from build123d import *

# Parameters (mm, degrees)
F0_R      = 26.924
F1_DEPTH  = 16.764
F0_R_2    = 27.94
F2_DEPTH  = 16.002
F0_R_3    = 22.225
F3_DEPTH  = 5.08
F4_SIZE   = 1.016
F0_W      = 3.175
F0_H      = 1.016
F5_DEPTH  = 23.622
F7_DEPTH  = 1.5875
F8_COUNT  = 3
F9_COUNT  = 2
F9_ANGLE  = 30
F10_COUNT = 3


with BuildPart() as f1:
    # F0 (on Top) → F1 (new body)
    with BuildSketch(Plane.XY):
        Circle(F0_R)
        with BuildLine():
            ThreePointArc((1.5875, 25.3503420835), (18.5132722661, 17.3901912008), (25.4, 0))
            ThreePointArc((25.4, 0), (-17.3901912008, -18.5132722661), (-1.5875, 25.3503420835))
            Line((-1.5875, 25.3503420835), (-1.5875, 25.908))
            Line((-1.5875, 25.908), (1.5875, 25.908))
            Line((1.5875, 25.908), (1.5875, 25.3503420835))
        make_face(mode=Mode.SUBTRACT)
        with BuildLine():
            ThreePointArc((-1.5875, 25.3503420835), (0, 25.4), (1.5875, 25.3503420835))
            Line((1.5875, 25.3503420835), (1.5875, 25.908))
            Line((1.5875, 25.908), (-1.5875, 25.908))
            Line((-1.5875, 25.908), (-1.5875, 25.3503420835))
        make_face()
    extrude(amount=F1_DEPTH)

    # F0 (on Top) → F2 (join)
    with BuildSketch(Plane.XY):
        Circle(F0_R_2)
        Circle(F0_R, mode=Mode.SUBTRACT)
    extrude(amount=F2_DEPTH)

    # F0 (on Top) → F3 (join)
    with BuildSketch(Plane.XY):
        with BuildLine():
            Line((1.5875, 24.892), (1.5875, 25.3503420835))
            ThreePointArc((1.5875, 25.3503420835), (0, 25.4), (-1.5875, 25.3503420835))
            Line((-1.5875, 25.3503420835), (-1.5875, 24.892))
            Line((-1.5875, 24.892), (1.5875, 24.892))
        make_face()
        with BuildLine():
            ThreePointArc((-1.5875, 25.3503420835), (-17.3901912008, -18.5132722661), (25.4, 0))
            ThreePointArc((25.4, 0), (18.5132722661, 17.3901912008), (1.5875, 25.3503420835))
            Line((1.5875, 25.3503420835), (1.5875, 24.892))
            Line((1.5875, 24.892), (1.5875, 23.876))
            Line((1.5875, 23.876), (-1.5875, 23.876))
            Line((-1.5875, 23.876), (-1.5875, 24.892))
            Line((-1.5875, 24.892), (-1.5875, 25.3503420835))
        make_face()
        Circle(F0_R_3, mode=Mode.SUBTRACT)
    extrude(amount=F3_DEPTH)

    # F4
    f4_edges = [f1.edges().sort_by_distance(p)[0] for p in [
        (-27.94, 0, 0),
        (-22.225, 0, 0),
    ]]
    chamfer(f4_edges, length=F4_SIZE)

    # F0 (on Top) → F5 (join)
    with BuildSketch(Plane.XY):
        with BuildLine():
            ThreePointArc((-1.5875, 25.3503420835), (0, 25.4), (1.5875, 25.3503420835))
            Line((1.5875, 25.3503420835), (1.5875, 25.908))
            Line((1.5875, 25.908), (-1.5875, 25.908))
            Line((-1.5875, 25.908), (-1.5875, 25.3503420835))
        make_face()
        with BuildLine():
            Line((1.5875, 24.892), (1.5875, 25.3503420835))
            ThreePointArc((1.5875, 25.3503420835), (0, 25.4), (-1.5875, 25.3503420835))
            Line((-1.5875, 25.3503420835), (-1.5875, 24.892))
            Line((-1.5875, 24.892), (1.5875, 24.892))
        make_face()
        with Locations((0, 24.384)):
            Rectangle(F0_W, F0_H)
    extrude(amount=F5_DEPTH)

    # F6 (on Right) → F7 (join, symmetric)
    with BuildSketch(Plane.YZ):
        Polygon((25.908, 20.8915), (27.94, 20.8915), (25.908, 23.622), align=None)
    extrude(amount=F7_DEPTH, both=True)

    # F8: F1 ×3 about axis
    f8_axis = Axis((0, 0, 10.7297506183), (0, 0, 1))


with BuildPart() as f1_1:
    add(f1.part)
    for i in range(1, F8_COUNT):
        add(f1.part.rotate(f8_axis, i * 360 / F8_COUNT))

    # F9: F1 ×2 about axis
    f9_axis = Axis((0, 0, 10.7297506183), (0, 0, 1))


with BuildPart() as f1_2:
    add(f1_1.part)
    for i in range(1, F9_COUNT):
        add(f1_1.part.rotate(f9_axis, i * F9_ANGLE / (F9_COUNT - 1)))

    # F10: F1 ×3 about axis
    f10_axis = Axis((0, 0, 10.7297506183), (0, 0, 1))


with BuildPart() as f1_3:
    add(f1_2.part)
    for i in range(1, F10_COUNT):
        add(f1_2.part.rotate(f10_axis, i * 360 / F10_COUNT))


solid = f1_3.part
Can you work these out from the model? Positions are in its coordinate system, mm. A direction names the side the tool comes from. Give positions to 0.01 mm unless a question says otherwise; leave off trailing zeros. Order: outer loops, then holes, each group sorted by start corner. A loop starts at its lowest first (then second) coordinate and runs counter-clockwise, first axis right, second up. Notation, with made-up numbers: (50.5, 44.25) - (64.5, 44.25) arc R31 ccw to (64.5, 73.25) - close; hole circle Ø8 at (-30, -28). An arc over 180 degrees is marked (long way). Write each question's results on one line, items separated by ' | '.
1) Please list where these lines run through material, in increasing order: line 1 along Y through (x, z) = (0, 4.35) (3 decimals); line 2 along X through (y, z) = (20, 9.25); line 3 along Z through (x, y) = (21.5, 15). Write a range as [from, to].
Final values:
line 1: y = [-27.94, -22.225], [22.225, 27.94] | line 2: x = [-19.51, -15.66], [-13.38, -13.11], [15.66, 19.51] | line 3: z = [0, 16.76]
2) If we mould it in two halves opening along Y, with no side actions, what happens to faces 1 (the face through (23, -13, 20.892)), 2 (the face through (-22.45, -12.93, 18.8)), 3 (the face through (-0.1, -22.5, 5.08))? For each: pulls with the +Y half, pulls with the -Y half, needs draft (parallel to the pull), parting line crosses it, or undercut.
Final values:
face 1: needs draft | face 2: pulls with the -Y half | face 3: undercut
3) Suppose I cut it at B-B, the plane z = 18.25. Write out the boundary of the cut face in (x, y).
Final values:
outline: (-23.23, -11.58) - (-21.64, -14.33) - (-19.88, -13.31) - (-21.47, -10.56) - close; (-14.33, -21.64) - (-11.58, -23.23) - (-10.56, -21.47) - (-13.31, -19.88) - close; (-14.33, 21.64) - (-13.31, 19.88) - (-10.56, 21.47) - (-11.58, 23.23) - close; (-1.59, 23.88) - (1.59, 23.88) - (1.59, 25.91) - (-1.59, 25.91) - close; (19.88, -13.31) - (21.64, -14.33) - (23.23, -11.58) - (21.47, -10.56) - close; (23.88, -1.59) - (25.91, -1.59) - (25.91, 1.59) - (23.88, 1.59) - close
4) On a 3-axis mill with a long thin cutter (end or side, diameter ignored), from which of +Z, -Z, +X, -X, +Y, -Y can I reach the whole of each face in a straight line? I mean faces 4 (the face through (21.199, 6.676, 3.02)), 5 (the face through (-11.1, 22.4, 16.5)). Say none if no direction works.
Final values:
face 4: +Z, -Z | face 5: +Z
5) Suppose I cut it at D-D, the plane z = 15. Write out the boundary of the cut face in (x, y), then the cut area to 3 significant figures.
Final values:
outline: circle Ø55.88 at (0, 0); hole (-22.75, -11.3) - (-21.47, -10.56) - (-19.88, -13.31) - (-21.16, -14.05) arc R25.4 ccw to (-14.05, -21.16) - (-13.31, -19.88) - (-10.56, -21.47) - (-11.3, -22.75) arc R25.4 ccw to (21.16, -14.05) - (19.88, -13.31) - (21.47, -10.56) - (22.75, -11.3) arc R25.4 ccw to (25.35, -1.59) - (23.88, -1.59) - (23.88, 1.59) - (25.35, 1.59) arc R25.4 ccw to (1.59, 25.35) - (1.59, 23.88) - (-1.59, 23.88) - (-1.59, 25.35) arc R25.4 ccw to (-11.3, 22.75) - (-10.56, 21.47) - (-13.31, 19.88) - (-14.05, 21.16) arc R25.4 ccw to start | area: 454 mm^2
6) Suppose I cut it at A-A, the plane x = 0. Write out the boundary of the cut face in (y, z) (1 decimal).
Final values:
outline: (-27.9, 1) - (-26.9, 0) - (-23.2, 0) - (-22.2, 1) - (-22.2, 5.1) - (-25.4, 5.1) - (-25.4, 16.8) - (-26.9, 16.8) - (-26.9, 16) - (-27.9, 16) - close; (22.2, 1) - (23.2, 0) - (26.9, 0) - (27.9, 1) - (27.9, 16) - (26.9, 16) - (26.9, 16.8) - (25.9, 16.8) - (25.9, 20.9) - (27.9, 20.9) - (25.9, 23.6) - (23.9, 23.6) - (23.9, 5.1) - (22.2, 5.1) - close
7) I'm going to push flat-ended pins straight in: pin 1 Ø8 at (y, z) = (-2, 15) entering from +X; pin 2 Ø5 at (y, z) = (-19.5, 20.5) entering from +X; pin 3 Ø2 at (y, z) = (26, 10.5) entering from +X; pin 4 Ø1 at (x, z) = (9.5, 5) entering from +Y. Where does each tip first touch, or does it pass through?
Final values:
pin 1: stops at x = 27.94 | pin 2: stops at x = -10.56 | pin 3: stops at x = 12.48 | pin 4: stops at y = 26.45
